Read the model definition and answer for the solid it produces. Units are mm, in the model's axes. A direction names the side the tool comes from. Coordinates: 2 decimals unless noted, no trailing zeros. Write each loop counter-clockwise with the first axis right and the second up, starting at its lowest first coordinate (ties: lowest second). Pieces come first, ordered by that corner, then holes.
from build123d import *

# Parameters (mm, degrees)
SKETCH1_R           = 15
BOSS_EXTRUDE1_DEPTH = 12
SKETCH2_R           = 9.5
BOSS_EXTRUDE2_DEPTH = 10
SKETCH3_R           = 5
CUT_EXTRUDE1_DEPTH  = 3
SKETCH4_R           = 1
BOSS_EXTRUDE3_DEPTH = 12


with BuildPart() as part:
    # Sketch1 → Boss-Extrude1 (new body)
    with BuildSketch(Plane(origin=(0, 0, 0), x_dir=(1, 0, 0), z_dir=(0, 1, 0))):
        with Locations(Location((0, 0, 0), (0, 0, 270))):
            Circle(SKETCH1_R)
    extrude(amount=BOSS_EXTRUDE1_DEPTH)

    # Sketch2 → Boss-Extrude2 (add)
    with BuildSketch(Plane(origin=(0, 12, 0), x_dir=(1, 0, 0), z_dir=(0, 1, 0))):
        with Locations(Location((0, 0, 0), (0, 0, 270))):
            Circle(SKETCH2_R)
    extrude(amount=BOSS_EXTRUDE2_DEPTH)

    # Sketch3 → Cut-Extrude1 (cut)
    with BuildSketch(Plane(origin=(0, 22, 0), x_dir=(1, 0, 0), z_dir=(0, 1, 0))):
        with Locations(Location((0, 0, 0), (0, 0, 270))):
            Circle(SKETCH3_R)
    extrude(amount=-CUT_EXTRUDE1_DEPTH, mode=Mode.SUBTRACT)

    # Sketch4 → Boss-Extrude3 (add)
    with BuildSketch(Plane.XZ):
        with Locations((15, 0)):
            Circle(SKETCH4_R)
        with Locations((7.5, -12.990381057)):
            Circle(SKETCH4_R)
        with Locations((-7.5, -12.990381057)):
            Circle(SKETCH4_R)
        with Locations((-15, 0)):
            Circle(SKETCH4_R)
        with Locations((-7.5, 12.990381057)):
            Circle(SKETCH4_R)
        with Locations((7.5, 12.990381057)):
            Circle(SKETCH4_R)
    extrude(amount=-BOSS_EXTRUDE3_DEPTH)


solid = part.part
Item 1: Find the intervals of material crossed by probe 1 along X at (y, z) = (20.2, 0); probe 2 along Y at (x, z) = (12.5, 0); probe 3 along Z at (x, y) = (-7.5, 1.5), in increasing order.
Item 2: The part is cut by section C-C (y = 9.5). Give the vertices of the cut face in (x, z).
Item 3: Determine the mould class of faces 3 (the cylindrical face through (-12.942, 5.916, -7.583)), 4 (the flat face through (0, 0, 0)), 5 (the cylindrical face through (7.98, 5.916, -13.867)) for opening direction X: +X half, -X half, draft (parallel to the pull), parting line (faces both ways), or undercut.
Item 4: The part is cut by section B-B (x = -7.5). Give the vertices of the cut face in (y, z).
Item 5: The part is cut by section A-A (z = 0). Give the vertices of the cut face in (x, y), and give its area (3 significant figures).
Item 6: Given pin 1 (10 mm diameter, centred on x = -6, y = 5, fed in from -Z); pin 2 (4 mm diameter, centred on y = 14.5, z = 0.5, fed in from +X); pin 3 (1 mm diameter, centred on y = 18.5, z = -4, fed in from -X); pin 4 (6 mm diameter, centred on x = 0, z = 0, fed in from -Y), each flat-ended and moving along its own axis, determine where each tip first touches the part or whether it passes through.
Item 7: The part is cut by section D-D (z = 8.75). Give the vertices of the cut face in (x, y).
Item 8: For faces 1 (the flat face through (-7, 12, 7)), 2 (the flat face through (-4, 22, 4)), determine the directions among +Z, -Z, +X, -X, +Y, -Y from which every point of the face is accessible in a straight line to the end or side of a thin tool.
Answer:
1. probe 1: x = -9.5 to -5, 5 to 9.5
1. probe 2: y = 0 to 12
1. probe 3: z = -13.99 to 13.99
2. outline: (-14.97, -1) arc R15 ccw to (-8.35, -12.46) arc R1 ccw (long way) to (-6.62, -13.46) arc R15 ccw to (6.62, -13.46) arc R1 ccw (long way) to (8.35, -12.46) arc R15 ccw to (14.97, -1) arc R1 ccw (long way) to (14.97, 1) arc R15 ccw to (8.35, 12.46) arc R1 ccw (long way) to (6.62, 13.46) arc R15 ccw to (-6.62, 13.46) arc R1 ccw (long way) to (-8.35, 12.46) arc R15 ccw to (-14.97, 1) arc R1 ccw (long way) to start
3. face 3: -X half
3. face 4: draft
3. face 5: undercut
4. outline: (0, -13.99) - (12, -13.99) - (12, -5.83) - (22, -5.83) - (22, 5.83) - (12, 5.83) - (12, 13.99) - (0, 13.99) - close
5. outline: (-16, 0) - (16, 0) - (16, 12) - (9.5, 12) - (9.5, 22) - (5, 22) - (5, 19) - (-5, 19) - (-5, 22) - (-9.5, 22) - (-9.5, 12) - (-16, 12) - close
5. area: 544 mm2
6. pin 1: stops at z = -14.97
6. pin 2: stops at x = 9.5
6. pin 3: stops at x = -8.83
6. pin 4: stops at y = 0
7. outline: (-12.18, 0) - (12.18, 0) - (12.18, 12) - (3.7, 12) - (3.7, 22) - (-3.7, 22) - (-3.7, 12) - (-12.18, 12) - close
8. face 1: +Y
8. face 2: +Z, -Z, +X, -X, +Y
